```python
from build123d import *

# Parameters (mm, degrees)
F1_DEPTH = 84
F2_W     = 61.5
F2_H     = 43.7
F3_DEPTH = 1.6


with BuildPart() as f1:
    # F0 (on Right) → F1 (new body)
    with BuildSketch(Plane.YZ):
        with BuildLine():
            Line((47.8, 20), (2.2, 20))
            ThreePointArc((2.2, 20), (0.644365, 19.355635), (0, 17.8))
            Line((0, 17.8), (0, 2.2))
            ThreePointArc((0, 2.2), (0.644365, 0.644365), (2.2, 0))
            Line((2.2, 0), (47.8, 0))
            ThreePointArc((47.8, 0), (49.355635, 0.644365), (50, 2.2))
            Line((50, 2.2), (50, 17.8))
            ThreePointArc((50, 17.8), (49.355635, 19.355635), (47.8, 20))
        make_face()
        with BuildLine():
            ThreePointArc((47.8, 18.4), (48.224264, 18.224264), (48.4, 17.8))
            Line((48.4, 17.8), (48.4, 2.2))
            ThreePointArc((48.4, 2.2), (48.224264, 1.775736), (47.8, 1.6))
            Line((47.8, 1.6), (2.2, 1.6))
            ThreePointArc((2.2, 1.6), (1.775736, 1.775736), (1.6, 2.2))
            Line((1.6, 2.2), (1.6, 17.8))
            ThreePointArc((1.6, 17.8), (1.775736, 18.224264), (2.2, 18.4))
            Line((2.2, 18.4), (47.8, 18.4))
        make_face(mode=Mode.SUBTRACT)
    extrude(amount=-F1_DEPTH)

    # F2 (on face) → F3 (cut, through all)
    with BuildSketch(Plane.XY.offset(20)):
        with Locations((-39.25, 25)):
            Rectangle(F2_W, F2_H)
    extrude(amount=-F3_DEPTH, mode=Mode.SUBTRACT)


solid = f1.part
```
Work out the finished part from the listing and answer in its coordinate system (mm). A direction names the side the tool comes from. Give positions to 0.01 mm unless a question says otherwise; leave off trailing zeros. Order: outer loops, then holes, each group sorted by start corner. A loop starts at its lowest first (then second) coordinate and runs counter-clockwise, first axis right, second up. Notation, with made-up numbers: (9, 78.25) - (39, 78.25) arc R34 cw to (39, 117.25) - close; hole circle Ø1 at (78.25, 83.5). An arc over 180 degrees is marked (long way). One line per item, written item: value. Start each with the question number.
1. For a pull along X with two mould halves and no side action, classify faces 1 (the face through (-8.5, 25, 19)), 2 (the face through (-41, 1.6, 10)), 3 (the face through (-84, 25, 1)) as released by +X, released by -X, zero draft, split by the parting line, or undercut.
2. Section C-C, the plane x = -30.5 is taken. Write down the section's boundary in (y, z).
3. Consider line 1 (Y direction, x = -26, z = 15.5); line 2 (Z direction, x = -7, y = 25.5); line 3 (Z direction, x = -36.5, y = 4). Determine where each line is inside the solid, lowest interval first.
4. Section B-B, the plane y = 21 is taken. Write down the section's boundary in (x, z), then the cut area to 3 significant figures.
5. Section A-A, the plane z = 4.5 is taken. Write down the section's boundary in (x, y).
6. Which of the six approach directions +Z, -Z, +X, -X, +Y, -Y give full straight-line access (tool end or side, diameter ignored) to faces 4 (the face through (-41, 0, 10)), 5 (the face through (-40, 3.15, 19)), 6 (the face through (-41, 48.4, 10))?
7. Section D-D, the plane x = -74 is taken. Write down the section's boundary in (y, z), then the cut area to 3 significant figures.
8. Each of these flat-tipped pins is pushed along its axis until it touches: pin 1 Ø13.5 at (x, y) = (-41.5, 18) entering from +Z; pin 2 Ø1.8 at (x, z) = (-25, 19.5) entering from -Y; pin 3 Ø1.3 at (x, z) = (-40.5, 19) entering from +Y; pin 4 Ø1.5 at (y, z) = (5, 16.5) entering from +X. Where does it stop, or does it pass through?
Filled sheet:
1. face 1: undercut
1. face 2: zero draft
1. face 3: released by -X
2. outline: (0, 2.2) arc R2.2 ccw to (2.2, 0) - (47.8, 0) arc R2.2 ccw to (50, 2.2) - (50, 17.8) arc R2.2 ccw to (47.8, 20) - (46.85, 20) - (46.85, 18.4) - (47.8, 18.4) arc R0.6 cw to (48.4, 17.8) - (48.4, 2.2) arc R0.6 cw to (47.8, 1.6) - (2.2, 1.6) arc R0.6 cw to (1.6, 2.2) - (1.6, 17.8) arc R0.6 cw to (2.2, 18.4) - (3.15, 18.4) - (3.15, 20) - (2.2, 20) arc R2.2 ccw to (0, 17.8) - close
3. line 1: 0 to 1.6, 48.4 to 50
3. line 2: 0 to 1.6, 18.4 to 20
3. line 3: 0 to 1.6
4. outline: (-84, 0) - (0, 0) - (0, 1.6) - (-84, 1.6) - close; (-84, 18.4) - (-70, 18.4) - (-70, 20) - (-84, 20) - close; (-8.5, 18.4) - (0, 18.4) - (0, 20) - (-8.5, 20) - close
4. area: 170 mm²
5. outline: (-84, 0) - (0, 0) - (0, 1.6) - (-84, 1.6) - close; (-84, 48.4) - (0, 48.4) - (0, 50) - (-84, 50) - close
6. face 4: +Z, -Z, +X, -X, -Y
6. face 5: +Z
6. face 6: +X, -X
7. outline: (0, 2.2) arc R2.2 ccw to (2.2, 0) - (47.8, 0) arc R2.2 ccw to (50, 2.2) - (50, 17.8) arc R2.2 ccw to (47.8, 20) - (2.2, 20) arc R2.2 ccw to (0, 17.8) - close; hole (1.6, 2.2) arc R0.6 ccw to (2.2, 1.6) - (47.8, 1.6) arc R0.6 ccw to (48.4, 2.2) - (48.4, 17.8) arc R0.6 ccw to (47.8, 18.4) - (2.2, 18.4) arc R0.6 ccw to (1.6, 17.8) - close
7. area: 210 mm²
8. pin 1: z = 1.6
8. pin 2: y = 0.15
8. pin 3: y = 49.93
8. pin 4: through
